from build123d import *

# Parameters (mm, degrees)
SKETCH1_W                 = 714.375
SKETCH1_H                 = 501.65
BOSS_EXTRUDE1_DEPTH       = 6.35
SKETCH2_R                 = 2.15265
CUT_EXTRUDE1_DEPTH        = 7.35
BOSS_EXTRUDE2_START       = -467.29015
SKETCH4_W                 = 714.375
SKETCH4_H                 = 6.35
BOSS_EXTRUDE2_DEPTH       = 432.9303
F_8_CLEARANCE_HOLE1_D     = 4.3053
F_8_CLEARANCE_HOLE1_DEPTH = 74.422
F_8_CLEARANCE_HOLE1_TIP   = 1.293442612
F_8_CLEARANCE_HOLE2_D     = 4.3053
F_8_CLEARANCE_HOLE2_DEPTH = 74.422
F_8_CLEARANCE_HOLE2_TIP   = 1.293442612
SKETCH11_R                = 12.7
CUT_EXTRUDE4_DEPTH        = 83.82
F_6_CLEARANCE_HOLE1_D     = 3.7973
F_6_CLEARANCE_HOLE1_DEPTH = 74.422
F_6_CLEARANCE_HOLE1_TIP   = 1.140824014
SKETCH14_R                = 1.778
SKETCH14_R_2              = 1.779075966
CUT_EXTRUDE5_DEPTH        = 7.62
SKETCH15_R                = 2.15265
CUT_EXTRUDE6_DEPTH        = 6.35


with BuildPart() as part:
    # Sketch1 → Boss-Extrude1 (new body)
    with BuildSketch(Plane(origin=(0, 0, 0), x_dir=(1, 0, 0), z_dir=(0, 1, 0))):
        Rectangle(SKETCH1_W, SKETCH1_H)
    extrude(amount=BOSS_EXTRUDE1_DEPTH)

    # Sketch2 → Cut-Extrude1 (cut, through all)
    with BuildSketch(Plane(origin=(0, 6.35, 0), x_dir=(1, 0, 0), z_dir=(0, 1, 0))):
        with Locations((-114.3, -214.3125)):
            Circle(SKETCH2_R)
        with Locations((-228.6, -214.3125)):
            Circle(SKETCH2_R)
        with Locations((228.6, -214.3125)):
            Circle(SKETCH2_R)
        with Locations((114.3, -214.3125)):
            Circle(SKETCH2_R)
        with Locations((114.3, 214.3125)):
            Circle(SKETCH2_R)
        with Locations((228.6, 214.3125)):
            Circle(SKETCH2_R)
        with Locations((-228.6, 214.3125)):
            Circle(SKETCH2_R)
        with Locations((-114.3, 214.3125)):
            Circle(SKETCH2_R)
    extrude(amount=-CUT_EXTRUDE1_DEPTH, mode=Mode.SUBTRACT)

    # Sketch4 → Boss-Extrude2 (add)
    with BuildSketch(Plane.XY.offset(250.825).offset(BOSS_EXTRUDE2_START)):
        with Locations((0, 3.175)):
            Rectangle(SKETCH4_W, SKETCH4_H)
    extrude(amount=BOSS_EXTRUDE2_DEPTH)

    # #8 Clearance Hole1
    with Locations(Plane(origin=(0, 6.35, 0), x_dir=(1, 0, 0), z_dir=(0, 1, 0))):
        with Locations((-273.3675, 231.775), (-136.2075, 231.775), (136.2075, 231.775), (273.3675, 231.775), (273.3675, 200.025), (136.2075, 200.025), (-136.2075, 200.025), (-273.3675, 200.025), (-273.3675, -200.025), (-273.3675, -231.775), (-136.2075, -231.775), (-136.2075, -200.025), (136.2075, -200.025), (136.2075, -231.775), (273.3675, -231.775), (273.3675, -200.025)):
            Hole(F_8_CLEARANCE_HOLE1_D / 2, depth=F_8_CLEARANCE_HOLE1_DEPTH)
            with Locations((0, 0, -(F_8_CLEARANCE_HOLE1_DEPTH + F_8_CLEARANCE_HOLE1_TIP / 2))):  # 118° drill point
                Cone(0, F_8_CLEARANCE_HOLE1_D / 2, F_8_CLEARANCE_HOLE1_TIP, mode=Mode.SUBTRACT)

    # #8 Clearance Hole2
    with Locations(Plane(origin=(0, 6.35, 0), x_dir=(1, 0, 0), z_dir=(0, 1, 0))):
        with Locations((-313.309, 231.93248), (313.309, 231.93248), (313.309, -231.93248), (-313.309, -231.93248)):
            Hole(F_8_CLEARANCE_HOLE2_D / 2, depth=F_8_CLEARANCE_HOLE2_DEPTH)
            with Locations((0, 0, -(F_8_CLEARANCE_HOLE2_DEPTH + F_8_CLEARANCE_HOLE2_TIP / 2))):  # 118° drill point
                Cone(0, F_8_CLEARANCE_HOLE2_D / 2, F_8_CLEARANCE_HOLE2_TIP, mode=Mode.SUBTRACT)

    # Sketch11 → Cut-Extrude4 (cut)
    with BuildSketch(Plane(origin=(0, 6.35, 0), x_dir=(1, 0, 0), z_dir=(0, 1, 0))):
        with Locations((204.7875, 0)):
            Circle(SKETCH11_R)
    extrude(amount=-CUT_EXTRUDE4_DEPTH, mode=Mode.SUBTRACT)

    # #6 Clearance Hole1
    with Locations(Plane(origin=(0, 6.35, 0), x_dir=(1, 0, 0), z_dir=(0, 1, 0))):
        with Locations((-349.1357, 196.07911), (-349.1357, 184.92089), (-349.1357, -184.92089), (-349.1357, -196.07911)):
            Hole(F_6_CLEARANCE_HOLE1_D / 2, depth=F_6_CLEARANCE_HOLE1_DEPTH)
            with Locations((0, 0, -(F_6_CLEARANCE_HOLE1_DEPTH + F_6_CLEARANCE_HOLE1_TIP / 2))):  # 118° drill point
                Cone(0, F_6_CLEARANCE_HOLE1_D / 2, F_6_CLEARANCE_HOLE1_TIP, mode=Mode.SUBTRACT)

    # Sketch14 → Cut-Extrude5 (cut)
    with BuildSketch(Plane.XZ):
        with Locations((-44.331384182, 202.954384182)):
            Circle(SKETCH14_R)
        with Locations((-17.390615818, 202.954384182)):
            Circle(SKETCH14_R)
        with Locations((-17.390615818, 176.013615818)):
            Circle(SKETCH14_R)
        with Locations((-44.331384182, 176.013615818)):
            Circle(SKETCH14_R)
        with Locations((124.912884182, 115.768884182)):
            Circle(SKETCH14_R)
        with Locations((124.91212, 88.82888)):
            Circle(SKETCH14_R_2)
        with Locations((97.972115818, 88.828115818)):
            Circle(SKETCH14_R)
        with Locations((97.972115818, 115.768884182)):
            Circle(SKETCH14_R)
        with Locations((97.972115818, -88.828115818)):
            Circle(SKETCH14_R)
        with Locations((124.912884182, -88.828115818)):
            Circle(SKETCH14_R)
        with Locations((124.912884182, -115.768884182)):
            Circle(SKETCH14_R)
        with Locations((97.972115818, -115.768884182)):
            Circle(SKETCH14_R)
        with Locations((-44.331384182, -176.013615818)):
            Circle(SKETCH14_R)
        with Locations((-17.390615818, -176.013615818)):
            Circle(SKETCH14_R)
        with Locations((-17.390615818, -202.954384182)):
            Circle(SKETCH14_R)
        with Locations((-44.331384182, -202.954384182)):
            Circle(SKETCH14_R)
    extrude(amount=-CUT_EXTRUDE5_DEPTH, mode=Mode.SUBTRACT)

    # Sketch15 → Cut-Extrude6 (cut)
    with BuildSketch(Plane(origin=(0, 6.35, 0), x_dir=(1, 0, 0), z_dir=(0, 1, 0))):
        with Locations((-262.509, 231.93375)):
            Circle(SKETCH15_R)
        with Locations((262.509, 231.93375)):
            Circle(SKETCH15_R)
        with Locations((262.509, -231.93375)):
            Circle(SKETCH15_R)
        with Locations((-262.509, -231.93375)):
            Circle(SKETCH15_R)
    extrude(amount=-CUT_EXTRUDE6_DEPTH, mode=Mode.SUBTRACT)


solid = part.part
Input: part model. Units: mm. Frame: model coordinates. Give positions to 0.01 mm unless a question says otherwise; leave off trailing zeros. Order: outer loops, then holes, each group sorted by start corner. A loop starts at its lowest first (then second) coordinate and runs counter-clockwise, first axis right, second up. Notation, with made-up numbers: (-28.5, -7) - (27.5, -7) arc R9 ccw to (27.5, 3) - close; hole circle Ø8 at (-15.5, -6). An arc over 180 degrees is marked (long way). Answer as a JSON object with one key per item and string values. Group by question number.
Q1. First-contact query: pin 1 Ø3.5 at (x, z) = (-262.51, -231.93) entering from +Y. Flat tip, straight axial feed; report the tip coordinate or a pass-through.
Q2. Mould query, pull axis X, two halves, no side actions, for faces 1 (the face through (-5, 6.35, -4)), 2 (the face through (216.901, 3.219, -3.815)). Classes: pulls with the +X half, pulls with the -X half, needs draft (parallel to the pull), parting line crosses it, or undercut.
Q3. Cut plane A-A, the plane z = 0. Output: boundary loops of the cut face in (x, y), then the cut area to 4 significant figures.
Results:
{
 "1": {"pin 1": "through"},
 "2": {"face 1": "needs draft", "face 2": "undercut"},
 "3": {"outline": "(-357.19, 0) - (192.09, 0) - (192.09, 6.35) - (-357.19, 6.35) - close; (217.49, 0) - (357.19, 0) - (357.19, 6.35) - (217.49, 6.35) - close", "area": "4,375 mm^2"}
}
